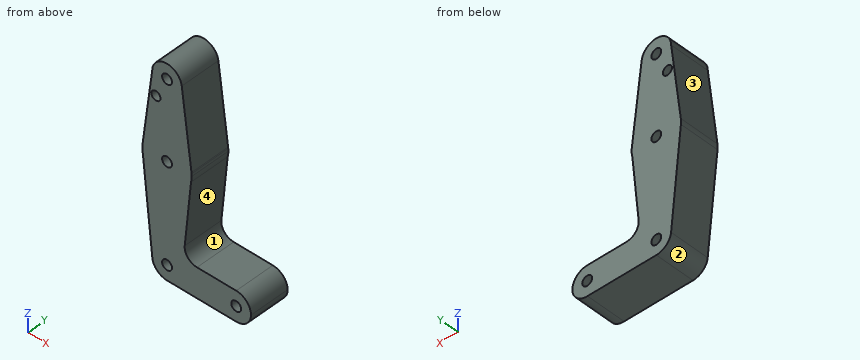
from build123d import *

# Parameters (mm, degrees)
F0_R     = 3.175
F0_R_2   = 2.938042
F1_DEPTH = 25.4


with BuildPart() as f1:
    # F0 (on Front) → F1 (new body)
    with BuildSketch(Plane.XZ):
        with BuildLine():
            ThreePointArc((0, -9.525), (6.735192, -6.735192), (9.525, 0))
            ThreePointArc((9.525, 0), (-0.476848, 9.513056), (-9.477255, -0.9525))
            ThreePointArc((-9.477255, -0.9525), (-6.389564, -7.063929), (0, -9.525))
        make_face()
        Circle(F0_R, mode=Mode.SUBTRACT)
        with BuildLine():
            ThreePointArc((-9.477255, -0.9525), (-0.476848, 9.513056), (9.525, 0))
            ThreePointArc((9.525, 0), (6.735192, -6.735192), (0, -9.525))
            Line((0, -9.525), (44.244344, -9.52278))
            ThreePointArc((44.244344, -9.52278), (34.925555, 0.102834), (44.45, 9.525))
            Line((44.45, 9.525), (19.271431, 9.525254))
            ThreePointArc((19.271431, 9.525254), (13.382074, 12.135023), (11.359216, 18.25086))
            Line((11.359216, 18.25086), (15.426409, 59.752799))
            ThreePointArc((15.426409, 59.752799), (-1.0955, 47.662844), (-15.795426, 61.9125))
            Line((-15.795426, 61.9125), (-9.477255, -0.9525))
        make_face()
        with BuildLine():
            ThreePointArc((-15.747457, 65.508289), (-15.873588, 63.711757), (-15.795426, 61.9125))
            ThreePointArc((-15.795426, 61.9125), (-1.0955, 47.662844), (15.426409, 59.752799))
            ThreePointArc((15.426409, 59.752799), (15.762453, 61.613022), (15.875, 63.5))
            ThreePointArc((15.875, 63.5), (15.854646, 64.303636), (15.793636, 65.105211))
            Line((15.793636, 65.105211), (15.698666, 65.859557))
            ThreePointArc((15.698666, 65.859557), (-0.17732, 79.37401), (-15.747457, 65.508289))
        make_face()
        with Locations((0, 63.5)):
            Circle(F0_R, mode=Mode.SUBTRACT)
        with BuildLine():
            ThreePointArc((44.45, 9.525), (34.925555, 0.102834), (44.244344, -9.52278))
            ThreePointArc((44.244344, -9.52278), (51.112085, -6.807514), (53.975, 0))
            ThreePointArc((53.975, 0), (51.185192, 6.735192), (44.45, 9.525))
        make_face()
        with Locations((44.45, 0)):
            Circle(F0_R, mode=Mode.SUBTRACT)
        with BuildLine():
            Line((-9.525, 114.3), (-15.747457, 65.508289))
            ThreePointArc((-15.747457, 65.508289), (-0.17732, 79.37401), (15.698666, 65.859557))
            Line((15.698666, 65.859557), (9.4504, 115.489771))
            ThreePointArc((9.4504, 115.489771), (9.506332, 114.896054), (9.525, 114.3))
            ThreePointArc((9.525, 114.3), (0, 104.775), (-9.525, 114.3))
        make_face()
        with Locations((-7.148621, 100.0252)):
            Circle(F0_R_2, mode=Mode.SUBTRACT)
        with BuildLine():
            ThreePointArc((15.793636, 65.105211), (15.750667, 65.482952), (15.698666, 65.859557))
            Line((15.698666, 65.859557), (15.793636, 65.105211))
        make_face()
        with BuildLine():
            ThreePointArc((9.4504, 115.489771), (-0.596054, 123.806332), (-9.525, 114.3))
            ThreePointArc((-9.525, 114.3), (0, 104.775), (9.525, 114.3))
            ThreePointArc((9.525, 114.3), (9.506332, 114.896054), (9.4504, 115.489771))
        make_face()
        with Locations((0, 114.3)):
            Circle(F0_R, mode=Mode.SUBTRACT)
    extrude(amount=F1_DEPTH)


solid = f1.part
Design review of the part built by this model. Coordinates are the model's own, in mm. Face numbers are marked on the shaded views. Coordinates: 2 decimals unless noted, no trailing zeros. Loops run counter-clockwise (first coordinate to the right, second up) from the corner with the lowest first, then second, coordinate; pieces in that order, holes last. Notation, with made-up numbers: (75, -40) - (86, -40) arc R30 ccw to (86, -15) - close; hole circle Ø6 at (54, 35.5). An arc over 180 degrees is marked (long way). Use CSV: the item, a comma, the result in double quotes. Start each with the question number.
1. Add section B-B on y = -10.75. Count the separate pieces of the cut face and the enclosed holes in it, plus the area to 3 significant figures.
2. Add section C-C on z = 87. Give the boundary of the cut face in (x, y), plus the area to 3 significant figures.
3. Add section A-A on x = 43. Give the boundary of the cut face in (y, z).
4. Clearance check with flat-ended pins moving along their axes: pin 1 (2 mm diameter, centred on x = 8, y = -9, fed in from +Z); pin 2 (5 mm diameter, centred on y = -5, z = 20, fed in from +X); pin 3 (1 mm diameter, centred on y = -17.5, z = 62, fed in from -X). State where each tip first meets the part, or that it passes through.
5. Add section D-D on x = 7.5. Give the boundary of the cut face in (y, z), plus the area to 3 significant figures.
6. Mouldability with a two-part tool opening along Z and no side actions: class the marked faces 1, 2, 3 and 4 as released by +Z, released by -Z, zero draft, split by the parting line, or undercut.
7. To check wall thickness, follow probe 1 along Z at (x, y) = (0, -7.5) (3 decimals); probe 2 along Z at (x, y) = (-1, -7); probe 3 along X at (y, z) = (-10.5, 115.5). State the ranges of each line that lie inside material, in increasing order.
Resolved:
1,separate pieces,"1"
1,enclosed holes,"5"
1,area,"3,890 mm2"
2,outline,"(-13.01, -25.4) - (13.04, -25.4) - (13.04, 0) - (-13.01, 0) - close"
2,area,"662 mm2"
3,outline,"(-25.4, -9.52) - (0, -9.52) - (0, -2.82) - (-25.4, -2.82) - close; (-25.4, 2.82) - (0, 2.82) - (0, 9.53) - (-25.4, 9.53) - close"
4,pin 1,"z = 120.76"
4,pin 2,"x = 11.78"
4,pin 3,"x = -15.84"
5,outline,"(-25.4, -9.52) - (0, -9.52) - (0, 120.17) - (-25.4, 120.17) - close"
5,area,"3,290 mm2"
6,face 1,"undercut"
6,face 2,"released by -Z"
6,face 3,"released by +Z"
6,face 4,"undercut"
7,probe 1,"-9.525 to -3.175, 3.175 to 60.325, 66.675 to 111.125, 117.475 to 123.825"
7,probe 2,"-9.47 to -3.01, 3.01 to 60.49, 66.51 to 111.29, 117.31 to 123.77"
7,probe 3,"-9.45 to -2.94, 2.94 to 9.45"
